Read the model definition and answer for the solid it produces. Units are mm, in the model's axes. Face numbers are marked on the shaded views. A direction names the side the tool comes from. Coordinates: 2 decimals unless noted, no trailing zeros. Loops run counter-clockwise (first coordinate to the right, second up) from the corner with the lowest first, then second, coordinate; pieces in that order, holes last. Notation, with made-up numbers: (37, 18.5) -> (72, 18.5) arc R12 cw to (72, 26.5) -> close; hole circle Ø7 at (66.25, 48.25). An arc over 180 degrees is marked (long way). Answer as CSV lines item,"result".
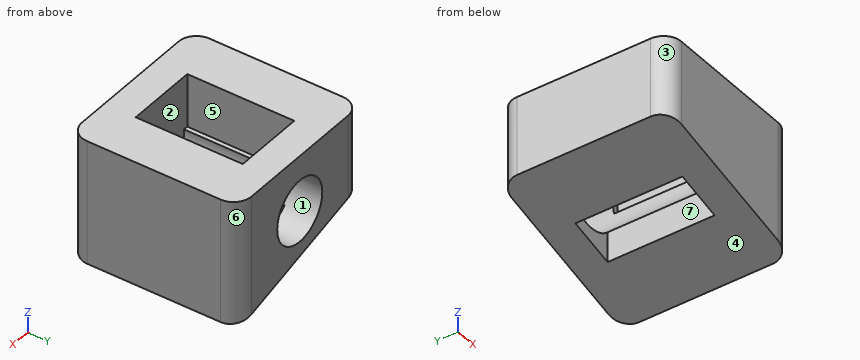
```python
from build123d import *

# Parameters (mm, degrees)
BOSS_EXTRUDE1_DEPTH = 10
CUT_EXTRUDE1_DEPTH  = 5
SKETCH11_W          = 9.5
SKETCH11_H          = 3
CUT_EXTRUDE9_DEPTH  = 15.588094461
SKETCH17_W          = 2.5
SKETCH17_H          = 6
CUT_EXTRUDE13_DEPTH = 10.701803956
CUT_EXTRUDE14_REACH = 14.721
SKETCH16_R          = 1.75
SKETCH18_W          = 4
SKETCH18_H          = 6
CUT_EXTRUDE15_DEPTH = 3


with BuildPart() as part:
    # Sketch1 → Boss-Extrude1 (new body)
    with BuildSketch(Plane.XY):
        with BuildLine():
            Line((-3.75, 4.75), (3.75, 4.75))
            ThreePointArc((3.75, 4.75), (4.457106781, 4.457106781), (4.75, 3.75))
            Line((4.75, 3.75), (4.75, -3.75))
            ThreePointArc((4.75, -3.75), (4.457106781, -4.457106781), (3.75, -4.75))
            Line((3.75, -4.75), (-3.75, -4.75))
            ThreePointArc((-3.75, -4.75), (-4.457106781, -4.457106781), (-4.75, -3.75))
            Line((-4.75, -3.75), (-4.75, 3.75))
            ThreePointArc((-4.75, 3.75), (-4.457106781, 4.457106781), (-3.75, 4.75))
        make_face()
    extrude(amount=BOSS_EXTRUDE1_DEPTH)

    # Sketch2 → Cut-Extrude1 (cut, symmetric)
    with BuildSketch(Plane(origin=(0, 0, 0), x_dir=(1, 0, 0), z_dir=(0, 1, 0))):
        Polygon((4.75, 0), (-4.75, 0), (-4.75, -2.545517328), align=None)
    extrude(amount=CUT_EXTRUDE1_DEPTH, both=True, mode=Mode.SUBTRACT)

    # Sketch11 → Cut-Extrude9 (cut, through all)
    with BuildSketch(Plane(origin=(0, 4.75, 0), x_dir=(1, 0, 0), z_dir=(0, 1, 0))):
        with Locations((0, -8.5)):
            Rectangle(SKETCH11_W, SKETCH11_H)
    extrude(amount=-CUT_EXTRUDE9_DEPTH, mode=Mode.SUBTRACT)

    # Sketch17 → Cut-Extrude13 (cut, through all)
    with BuildSketch(Plane.XY.offset(7)):
        Rectangle(SKETCH17_W, SKETCH17_H)
    extrude(amount=-CUT_EXTRUDE13_DEPTH, mode=Mode.SUBTRACT)

    # Cut-Extrude14: up to this face of the body (flat: up to its plane)
    cut_extrude14_end = Plane(part.part.faces().sort_by_distance((0.024367206, -3, 4.133114745))[0])
    # Sketch16 → Cut-Extrude14 (cut, up to the picked face)
    with BuildSketch(Plane(origin=(0, 4.75, 0), x_dir=(1, 0, 0), z_dir=(0, 1, 0)), mode=Mode.PRIVATE) as cut_extrude14_sk1:
        with Locations(Location((-0.002235874, -3.861548216, 0), (0, 0, 270))):
            Circle(SKETCH16_R)
    cut_extrude14_tool1 = split(extrude(cut_extrude14_sk1.sketch, amount=-CUT_EXTRUDE14_REACH, mode=Mode.PRIVATE), bisect_by=cut_extrude14_end, keep=Keep.BOTH, mode=Mode.PRIVATE)
    add(cut_extrude14_tool1.solids().sort_by(Axis((-0.002236, 4.75, 3.861548), (0, -1, 0)))[0], mode=Mode.SUBTRACT)

    # Sketch18 → Cut-Extrude15 (cut)
    with BuildSketch(Plane.XY.offset(7)):
        Rectangle(SKETCH18_W, SKETCH18_H)
    extrude(amount=-CUT_EXTRUDE15_DEPTH, mode=Mode.SUBTRACT)


solid = part.part
```
Q1. A cutting plane is placed at C-C, the plane x = 0.25. Write down the section's boundary in (y, z), and give its area (3 significant figures).
Results:
outline,"(-4.75, 1.21) -> (-3, 1.21) -> (-3, 7) -> (-4.75, 7) -> close; (3, 1.21) -> (4.75, 1.21) -> (4.75, 2.13) -> (3, 2.13) -> close; (3, 5.59) -> (4.75, 5.59) -> (4.75, 7) -> (3, 7) -> close"
area,"14.2 mm²"
Q2. Given pin 1 Ø1 at (x, y) = (1.5, -3.5) entering from -Z; pin 2 Ø3 at (x, z) = (0, 3.86) entering from +Y, each flat-ended and moving along its own axis, determine where each tip first touches the part or whether it passes through.
Results:
pin 1,"stops at z = 0.74"
pin 2,"stops at y = -3"
Q3. A cutting plane is placed at B-B, the plane z = 6.5. Write down the section's boundary in (x, y).
Results:
outline,"(-4.75, -3.75) arc R1 ccw to (-3.75, -4.75) -> (3.75, -4.75) arc R1 ccw to (4.75, -3.75) -> (4.75, 3.75) arc R1 ccw to (3.75, 4.75) -> (-3.75, 4.75) arc R1 ccw to (-4.75, 3.75) -> close; hole (-2, -3) -> (2, -3) -> (2, 3) -> (-2, 3) -> close"
Q4. For the marked faces 1, 2 and 3, determine the directions among +Z, -Z, +X, -X, +Y, -Y from which every point of the face is accessible in a straight line to the end or side of a thin tool.
Results:
face 1,"+Y"
face 2,"+Z"
face 3,"+Z, -Z, -X, -Y"
Q5. For a pull along Y with two mould halves and no side action, classify the marked faces 4, 5, 6 and 7 as pulls with the +Y half, pulls with the -Y half, needs draft (parallel to the pull), parting line crosses it, or undercut.
Results:
face 4,"needs draft"
face 5,"undercut"
face 6,"pulls with the +Y half"
face 7,"undercut"
Q6. Find the intervals of material crossed by probe 1 along Y at (x, z) = (0.5, 6.5); probe 2 along X at (y, z) = (1, 5.75); probe 3 along Y at (x, z) = (-1, 5.25), in increasing order. Write a range as [from, to].
Results:
probe 1,"y = [-4.75, -3], [3, 4.75]"
probe 2,"x = [-4.75, -2], [2, 4.75]"
probe 3,"y = [-4.75, -3]"
Q7. A cutting plane is placed at A-A, the plane y = 0.5. Write down the section's boundary in (x, z).
Results:
outline,"(-4.75, 2.55) -> (-1.25, 1.61) -> (-1.25, 2.63) arc R1.75 cw to (-1.75, 4) -> (-2, 4) -> (-2, 7) -> (-4.75, 7) -> close; (1.25, 0.94) -> (4.75, 0) -> (4.75, 7) -> (2, 7) -> (2, 4) -> (1.74, 4) arc R1.75 cw to (1.25, 2.64) -> close"
Q8. A cutting plane is placed at D-D, the plane z = 4.25. Write down the section's boundary in (x, y).
Results:
outline,"(-4.75, -3.75) arc R1 ccw to (-3.75, -4.75) -> (3.75, -4.75) arc R1 ccw to (4.75, -3.75) -> (4.75, 3.75) arc R1 ccw to (3.75, 4.75) -> (1.7, 4.75) -> (1.7, 3) -> (2, 3) -> (2, -3) -> (-2, -3) -> (-2, 3) -> (-1.71, 3) -> (-1.71, 4.75) -> (-3.75, 4.75) arc R1 ccw to (-4.75, 3.75) -> close"
